```python
from build123d import *

# Parameters (mm, degrees)
F1_DEPTH = 812.8
F2_W     = 323.85
F2_H     = 149.815533
F2_R     = 15.875
F2_W_2   = 203.2
F2_H_2   = 148.416346
F3_DEPTH = 25.4
F4_W     = 76.2
F4_H     = 419.1
F4_R     = 11.176
F5_DEPTH = 57.15
F6_W     = 152.4
F6_H     = 241.3
F6_R     = 7.14375
F7_DEPTH = 12.7


with BuildPart() as f1:
    # F0 (on Right) → F1 (new body, symmetric)
    with BuildSketch(Plane.YZ):
        with BuildLine():
            ThreePointArc((317.5, 31.75), (326.79936, 9.29936), (349.25, 0))
            Line((349.25, 0), (457.2, 0))
            Line((457.2, 0), (457.2, 12.7))
            Line((457.2, 12.7), (349.25, 12.7))
            ThreePointArc((349.25, 12.7), (335.779616, 18.279616), (330.2, 31.75))
            Line((330.2, 31.75), (330.2, 368.3))
            ThreePointArc((330.2, 368.3), (320.90064, 390.75064), (298.45, 400.05))
            Line((298.45, 400.05), (0, 400.05))
            Line((0, 400.05), (-298.45, 400.05))
            ThreePointArc((-298.45, 400.05), (-320.90064, 390.75064), (-330.2, 368.3))
            Line((-330.2, 368.3), (-330.2, 31.75))
            ThreePointArc((-330.2, 31.75), (-335.779616, 18.279616), (-349.25, 12.7))
            Line((-349.25, 12.7), (-457.2, 12.7))
            Line((-457.2, 12.7), (-457.2, 0))
            Line((-457.2, 0), (-349.25, 0))
            ThreePointArc((-349.25, 0), (-326.79936, 9.29936), (-317.5, 31.75))
            Line((-317.5, 31.75), (-317.5, 368.3))
            ThreePointArc((-317.5, 368.3), (-311.920384, 381.770384), (-298.45, 387.35))
            Line((-298.45, 387.35), (0, 387.35))
            Line((0, 387.35), (298.45, 387.35))
            ThreePointArc((298.45, 387.35), (311.920384, 381.770384), (317.5, 368.3))
            Line((317.5, 368.3), (317.5, 31.75))
        make_face()
    extrude(amount=F1_DEPTH, both=True)

    # F2 (on face) → F3 (join)
    with BuildSketch(Plane.XY.offset(400.05)):
        with Locations((-408.051, -234.850373)):
            Rectangle(F2_W, F2_H)
        with Locations((-474.726, -243.856796)):
            Circle(F2_R, mode=Mode.SUBTRACT)
        with Locations((147.574, -241.293997)):
            Rectangle(F2_W_2, F2_H_2)
        with Locations((154.178, -251.150241)):
            Circle(F2_R, mode=Mode.SUBTRACT)
        with Locations((-408.051, 234.850373)):
            Rectangle(F2_W, F2_H)
        with Locations((-474.726, 243.856796)):
            Circle(F2_R, mode=Mode.SUBTRACT)
        with Locations((147.574, 241.293997)):
            Rectangle(F2_W_2, F2_H_2)
        with Locations((154.178, 251.150241)):
            Circle(F2_R, mode=Mode.SUBTRACT)
    extrude(amount=F3_DEPTH)

    # F4 (on face) → F5 (join)
    with BuildSketch(Plane.XY.offset(400.05)):
        with Locations((547.624, 0)):
            Rectangle(F4_W, F4_H)
        with Locations((547.624, -146.05)):
            Circle(F4_R, mode=Mode.SUBTRACT)
        with Locations((547.624, 146.05)):
            Circle(F4_R, mode=Mode.SUBTRACT)
        with Locations((319.024, 0)):
            Rectangle(F4_W, F4_H)
        with Locations((319.024, -146.05)):
            Circle(F4_R, mode=Mode.SUBTRACT)
        with Locations((319.024, 146.05)):
            Circle(F4_R, mode=Mode.SUBTRACT)
    extrude(amount=F5_DEPTH)

    # F6 (on face) → F7 (join)
    with BuildSketch(Plane.XY.offset(400.05)):
        with Locations((720.598, 0)):
            Rectangle(F6_W, F6_H)
        with Locations((682.498, -63.5)):
            Circle(F6_R, mode=Mode.SUBTRACT)
        with Locations((758.698, -63.5)):
            Circle(F6_R, mode=Mode.SUBTRACT)
        with Locations((682.498, 63.5)):
            Circle(F6_R, mode=Mode.SUBTRACT)
        with Locations((758.698, 63.5)):
            Circle(F6_R, mode=Mode.SUBTRACT)
    extrude(amount=F7_DEPTH)


solid = f1.part
```
Verification items for the finished model (mm, model axes). A direction names the side the tool comes from. Coordinates: 2 decimals unless noted, no trailing zeros. Loops run counter-clockwise (first coordinate to the right, second up) from the corner with the lowest first, then second, coordinate; pieces in that order, holes last. Notation, with made-up numbers: (-31.75, 85) -> (-3.75, 85) arc R16 cw to (-3.75, 94) -> close; hole circle Ø8 at (-5, 72.25). An arc over 180 degrees is marked (long way). Put each result on its own line as item: value.
1. Thickness scan on line 1 (X direction, y = 184, z = 400.5); line 2 (Y direction, x = -663.5, z = 176); line 3 (Z direction, x = -320.5, y = -173). Record the ranges inside material, lowest first.
Result set:
line 1: x = -569.98 to -246.13, 45.97 to 249.17, 280.92 to 357.12, 509.52 to 585.72
line 2: y = -330.2 to -317.5, 317.5 to 330.2
line 3: z = 387.35 to 425.45
2. Mould release check, pull along Y, two halves, no side actions. Record for faces 1 (the face through (162.712, 264.536, 412.572)), 2 (the face through (11, -330.2, 202)), 3 (the face through (720, 2, 412.75)): pulls with the +Y half, pulls with the -Y half, needs draft (parallel to the pull), parting line crosses it, or undercut.
Result set:
face 1: undercut
face 2: pulls with the -Y half
face 3: needs draft
3. Section check B-B, the plane y = 21. Record the boundary of the cut face in (x, z).
Result set:
outline: (-812.8, 387.35) -> (812.8, 387.35) -> (812.8, 400.05) -> (796.8, 400.05) -> (796.8, 412.75) -> (644.4, 412.75) -> (644.4, 400.05) -> (585.72, 400.05) -> (585.72, 457.2) -> (509.52, 457.2) -> (509.52, 400.05) -> (357.12, 400.05) -> (357.12, 457.2) -> (280.92, 457.2) -> (280.92, 400.05) -> (-812.8, 400.05) -> close
4. Gauge pin test, flat ends, axial feed: P1, Ø4.5, axis at x = 684.5, y = 62, coming from the +Z side; P2, Ø1, axis at x = -173.5, y = -156.5, coming from the -Z side; P3, Ø12.5, axis at y = 218.5, z = 418.5, coming from the -X side. Record the tip position at first contact, or that the pin passes through.
Result set:
P1: stops at z = 400.05
P2: stops at z = 387.35
P3: stops at x = -569.98
5. Section check A-A, the plane z = 106. Record the boundary of the cut face in (x, y), then the cut area to 3 significant figures.
Result set:
outline: (-812.8, -330.2) -> (812.8, -330.2) -> (812.8, -317.5) -> (-812.8, -317.5) -> close; (-812.8, 317.5) -> (812.8, 317.5) -> (812.8, 330.2) -> (-812.8, 330.2) -> close
area: 41,300 mm^2
6. Section check C-C, the plane x = -689. Record the boundary of the cut face in (y, z), then the cut area to 3 significant figures.
Result set:
outline: (-457.2, 0) -> (-349.25, 0) arc R31.75 ccw to (-317.5, 31.75) -> (-317.5, 368.3) arc R19.05 cw to (-298.45, 387.35) -> (298.45, 387.35) arc R19.05 cw to (317.5, 368.3) -> (317.5, 31.75) arc R31.75 ccw to (349.25, 0) -> (457.2, 0) -> (457.2, 12.7) -> (349.25, 12.7) arc R19.05 cw to (330.2, 31.75) -> (330.2, 368.3) arc R31.75 ccw to (298.45, 400.05) -> (-298.45, 400.05) arc R31.75 ccw to (-330.2, 368.3) -> (-330.2, 31.75) arc R19.05 cw to (-349.25, 12.7) -> (-457.2, 12.7) -> close
area: 20,900 mm^2
7. Tool access check on faces 4 (the face through (146, 226, 425.45)), 5 (the face through (11, 330.2, 198)), 6 (the face through (318, -209.55, 428)), 7 (the face through (11, 317.5, 202)). Record the directions out of +Z, -Z, +X, -X, +Y, -Y that give a thin tool (end or side, any length) a straight path to the whole face; none if there is none.
Result set:
face 4: +Z, -X, +Y, -Y
face 5: +Z, +X, -X, +Y
face 6: +Z, +X, -Y
face 7: -Z, +X, -X
